Source: CAD feature listing. Evaluate the final solid. Frame: model axes, mm. Coordinates: 2 decimals unless noted, no trailing zeros. Order: outer loops, then holes, each group sorted by start corner. A loop starts at its lowest first (then second) coordinate and runs counter-clockwise, first axis right, second up.
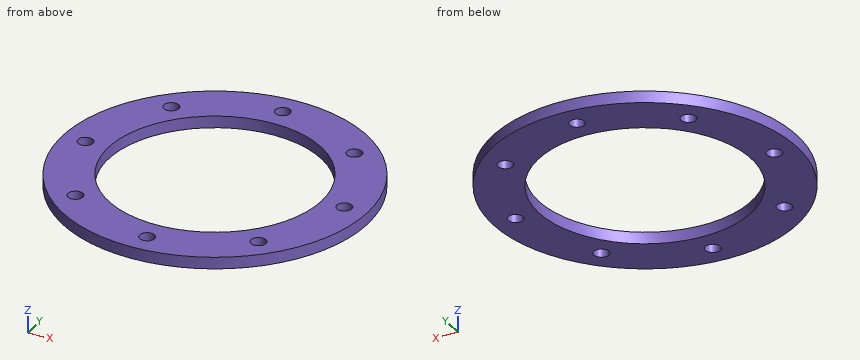
Autodesk Inventor part; units mm, degrees
ref_plane "YZ Plane" through (0, 0, 0) normal (1, 0, 0) x (0, 1, 0)
ref_plane "XZ Plane" through (0, 0, 0) normal (0, 1, 0) x (-1, 0, 0)
ref_plane "XY Plane" through (0, 0, 0) normal (0, 0, 1) x (1, 0, 0)
sketch "スケッチ1" plane through (0, 0, 0) normal (0, 0, 1) x (1, 0, 0)
  circle A0 centre (0, 46.1553) radius 11.5
  circle A1 centre (15, 0.6557) radius 1.6
  circle A2 centre (-15, 0.6557) radius 1.6
  circle A3 centre (15, -29.3443) radius 1.6
  circle A4 centre (15, -59.3443) radius 1.6
  circle A5 centre (-15, -29.3443) radius 1.6
  circle A6 centre (-15, -59.3443) radius 1.6
  circle A7 centre (13.5, 17.896) radius 1.1
  circle A8 centre (13.5, 44.896) radius 1.1
  circle A9 centre (-13.5, 17.896) radius 1.1
  circle A10 centre (-13.5, 44.896) radius 1.1
  line L0 (-22.5, 19.3457) -> (-22.5, -66.8443)
  line L1 (-22.5, -66.8443) -> (22.5, -66.8443)
  line L2 (22.5, -66.8443) -> (22.5, 19.3457)
  arc A11 (22.5, 19.3457) -> (-22.5, 19.3457) centre (0, 46.1553) ccw
  circle A12 centre (0, 46.1553) radius 5
  circle A13 centre (3.8451, 52.0046) radius 0.8
  circle A14 centre (6.855, 47.5725) radius 0.8
  circle A15 centre (5.8494, 42.3101) radius 0.8
  circle A16 centre (1.4172, 39.3002) radius 0.8
  circle A17 centre (-3.8451, 40.3059) radius 0.8
  circle A18 centre (-6.855, 44.738) radius 0.8
  circle A19 centre (-5.8494, 50.0004) radius 0.8
  circle A20 centre (-1.4172, 53.0103) radius 0.8
  circle A21 centre (0, 46.1553) radius 10
  circle A22 centre (0, 46.1553) radius 32.5
  circle A23 centre (0, 46.1553) radius 22.7
  circle A24 centre (0, 46.1553) radius 22.7 construction
  line L3 (0, 68.8553) -> (0, 78.6553) construction
  circle A25 centre (0, 73.7553) radius 1.6
  circle A26 centre (-19.5161, 65.6714) radius 1.6
  circle A27 centre (-27.6, 46.1553) radius 1.6
  circle A28 centre (-19.5161, 26.6391) radius 1.6
  circle A29 centre (0, 18.5553) radius 1.6
  circle A30 centre (19.5161, 26.6391) radius 1.6
  circle A31 centre (27.6, 46.1553) radius 1.6
  circle A32 centre (19.5161, 65.6714) radius 1.6
  circle A33 centre (0, 46.1553) radius 27.6 construction
  point P0 (0, 0)
  dimension "d0" = 65
  dimension "d1" = 45.4
  dimension "d3" = 3.2
  dimension "d6" = 360
  dimension "d13" = 27.6
  dimension "d14" = 55.2
extrude "押し出し1" add sketch "スケッチ1" along normal blind 2.5 contours A7 | A9 | A22
properties part number "軸受けワッシャA_ダブルスラスト用(t2_ジュラコン)" material "アルミニウム 6061"
Q1. Material intervals for line 1 along Y through (x, z) = (0, 1.7); line 2 along X through (y, z) = (67, 0.5); line 3 along Y through (x, z) = (20, 0.4), sorted ascending.
Solutions:
line 1: y = 13.66 to 16.96, 20.16 to 23.46, 68.86 to 72.16, 75.36 to 78.66
line 2: x = -24.93 to -20.41, -18.62 to -8.99, 8.99 to 18.62, 20.41 to 24.93
line 3: y = 20.54 to 25.11, 28.16 to 35.42, 56.89 to 64.15, 67.2 to 71.77
Q2. Pin query (flat end, axial travel): P1, Ø4, axis at x = 19.52, y = 26.64, coming from the -Z side. Return the tip coordinate at first contact, or that it passes through.
Solutions:
P1: stops at z = 0
Q3. Section query B-B on y = 29. Output: boundary loops of the cut face in (x, z).
Solutions:
outline: (-27.6, 0) - (-14.87, 0) - (-14.87, 2.5) - (-27.6, 2.5) - close; (14.87, 0) - (27.6, 0) - (27.6, 2.5) - (14.87, 2.5) - close
Q4. Section query D-D on z = 1.85. Give the number of separate pieces and of enclosed holes in the cut face, plus the area to 3 significant figures.
Solutions:
separate pieces: 1
enclosed holes: 9
area: 1,640 mm2
Q5. Section query A-A on x = 0. Output: boundary loops of the cut face in (y, z).
Solutions:
outline: (13.66, 0) - (16.96, 0) - (16.96, 2.5) - (13.66, 2.5) - close; (20.16, 0) - (23.46, 0) - (23.46, 2.5) - (20.16, 2.5) - close; (68.86, 0) - (72.16, 0) - (72.16, 2.5) - (68.86, 2.5) - close; (75.36, 0) - (78.66, 0) - (78.66, 2.5) - (75.36, 2.5) - close
Q6. Section query C-C on x = -7. Output: boundary loops of the cut face in (y, z), plus the area to 3 significant figures.
Solutions:
outline: (14.42, 0) - (24.56, 0) - (24.56, 2.5) - (14.42, 2.5) - close; (67.75, 0) - (77.89, 0) - (77.89, 2.5) - (67.75, 2.5) - close
area: 50.7 mm2
